```python
from build123d import *

# Parameters (mm, degrees)
EXTRUDE_1_DEPTH     = 20
CUT_EXTRUDE_3_DEPTH = 149.381528207
CUT_EXTRUDE_4_DEPTH = 154.011402085
CUT_EXTRUDE_5_DEPTH = 149.381528207
CUT_EXTRUDE_6_DEPTH = 142.921339686


with BuildPart() as part:
    # Эскиз1 → Бобышка-Вытянуть1 (new body)
    with BuildSketch(Plane.XY):
        Polygon((0, 0), (0, -8), (100, -8), (121.213203436, 13.213203436), (121.213203436, 83.213203436), (113.213203436, 83.213203436), (113.213203436, 16.526911935), (96.686291501, 0), align=None)
    extrude(amount=EXTRUDE_1_DEPTH)

    # Эскиз4 → Вырез-Вытянуть3 (cut, through all)
    with BuildSketch(Plane.ZY):
        Polygon((0, -8), (2.309401077, -4), (17.690598923, -4), (20, -8), align=None)
    extrude(amount=-CUT_EXTRUDE_3_DEPTH, mode=Mode.SUBTRACT)

    # Эскиз5 → Вырез-Вытянуть4 (cut, through all)
    with BuildSketch(Plane(origin=(0, 83.213203436, 0), x_dir=(1, 0, 0), z_dir=(0, 1, 0))):
        Polygon((121.213203436, 0), (117.213203436, -2.309401077), (117.213203436, -17.690598923), (121.213203436, -20), align=None)
    extrude(amount=-CUT_EXTRUDE_4_DEPTH, mode=Mode.SUBTRACT)

    # Эскиз6 → Вырез-Вытянуть5 (cut, through all)
    with BuildSketch(Plane(origin=(0, 0, 0), x_dir=(1, 0, 0), z_dir=(0, 1, 0))):
        with BuildLine():
            Line((7.870014132, -7.663568904), (84.104423022, -7.663568904))
            ThreePointArc((84.104423022, -7.663568904), (86.440854117, -10), (84.104423022, -12.336431096))
            Line((84.104423022, -12.336431096), (7.870014132, -12.336431096))
            ThreePointArc((7.870014132, -12.336431096), (5.533583037, -10), (7.870014132, -7.663568904))
        make_face()
    extrude(amount=-CUT_EXTRUDE_5_DEPTH, mode=Mode.SUBTRACT)

    # Эскиз7 → Вырез-Вытянуть6 (cut, through all)
    with BuildSketch(Plane.ZY.offset(-113.213203436)):
        with BuildLine():
            Line((12.340286207, 77.716506994), (12.340286207, 24.800035528))
            ThreePointArc((12.340286207, 24.800035528), (10, 22.45974932), (7.659713793, 24.800035528))
            Line((7.659713793, 24.800035528), (7.659713793, 77.716506994))
            ThreePointArc((7.659713793, 77.716506994), (10, 80.056793201), (12.340286207, 77.716506994))
        make_face()
    extrude(amount=-CUT_EXTRUDE_6_DEPTH, mode=Mode.SUBTRACT)


solid = part.part
```
The listing builds one solid part. Answer for the finished solid, in the listing's coordinates (mm). A direction names the side the tool comes from. Coordinates: 2 decimals unless noted, no trailing zeros. Write each loop counter-clockwise with the first axis right and the second up, starting at its lowest first coordinate (ties: lowest second). Pieces come first, ordered by that corner, then holes. Notation, with made-up numbers: M 17.25,10.5 L 39.25,10.5 A13 ccw 39.25,20.5 Z; hole C 1.5,75 d7. An arc over 180 degrees is marked long. Use a Markdown table: item, result. Add a question column.
1. Section C-C (x = 13.5) is taken. Give the vertices of the cut face in (y, z).
2. Which of the six approach directions +Z, -Z, +X, -X, +Y, -Y give full straight-line access (tool end or side, diameter ignored) to faces 1 (the flat face through (119.24, 46.73, 1.14)), 2 (the flat face through (51.27, -5.97, 18.83)), 3 (the flat face through (45, -2, 7.664))?
3. Given P1, Ø10, axis at x = 61.5, z = 5, coming from the +Y side; P2, Ø10, axis at y = 48.5, z = 12, coming from the -X side; P3, Ø1.5, axis at x = 16, z = 16.5, coming from the -Y side; P4, Ø3, axis at x = 28, y = -1.5, coming from the -Z side, each flat-ended and moving along its own axis, determine where each tip first touches the part or whether it passes through.
4. Section B-B (z = 10) is taken. Give the vertices of the cut face in (x, y), plus the area to 3 significant figures.
5. Section D-D (x = 98) is taken. Give the vertices of the cut face in (y, z), plus the area to 3 significant figures.
6. For a pull along Z with two mould halves and no side action, classify faces 4 (the flat face through (83, -3, 0)), 5 (the cylindrical face through (115.185, 80.056, 9.949)), 6 (the flat face through (110, 2, 10)) as +Z half, -Z half, draft (parallel to the pull), parting line (faces both ways), or undercut.
7. Straight lines are drawn through the part: line 1 along Z through (x, y) = (29.5, -2); line 2 along X through (y, z) = (36, 15.5); line 3 along Y through (x, z) = (7, 14.5). For each, find the intervals that lie inside material, in ascending order. Write a range as [from, to].
8. Section A-A (y = 43) is taken. Give the vertices of the cut face in (x, z).
Data:
| question | item | result |
|---|---|---|
| 1 | outline | M -8,0 L 0,0 L 0,7.66 L -4,7.66 L -4,2.31 Z; M -8,20 L -4,17.69 L -4,12.34 L 0,12.34 L 0,20 Z |
| 2 | face 1 | +X, +Y, -Y |
| 2 | face 2 | +X, -X, -Y |
| 2 | face 3 | +Y, -Y |
| 3 | P1 | stops at y = 0 |
| 3 | P2 | stops at x = 113.21 |
| 3 | P3 | stops at y = -4 |
| 3 | P4 | stops at z = 0 |
| 4 | outline | M 0,-4 L 5.53,-4 L 5.53,0 L 0,0 Z; M 86.44,-4 L 104,-4 L 117.21,9.21 L 117.21,22.46 L 113.21,22.46 L 113.21,16.53 L 96.69,0 L 86.44,0 Z; M 113.21,80.06 L 117.21,80.06 L 117.21,83.21 L 113.21,83.21 Z |
| 4 | area | 297 mm2 |
| 5 | outline | M -8,0 L 1.31,0 L 1.31,20 L -8,20 L -4,17.69 L -4,2.31 Z |
| 5 | area | 116 mm2 |
| 6 | face 4 | -Z half |
| 6 | face 5 | undercut |
| 6 | face 6 | draft |
| 7 | line 1 | z = [0, 7.66], [12.34, 20] |
| 7 | line 2 | x = [113.21, 117.21] |
| 7 | line 3 | y = [-4, 0] |
| 8 | outline | M 113.21,0 L 121.21,0 L 117.21,2.31 L 117.21,7.66 L 113.21,7.66 Z; M 113.21,12.34 L 117.21,12.34 L 117.21,17.69 L 121.21,20 L 113.21,20 Z |
